from build123d import *

# Parameters (mm, degrees)
SKETCH_1_W          = 56
SKETCH_1_H          = 36
SKETCH_1_R          = 1.6
EXTRUDE_1_DEPTH     = 3
FILLET_1_R          = 3
SKETCH_2_W          = 22
SKETCH_2_H          = 6
SKETCH_2_R          = 1.4
EXTRUDE_2_DEPTH     = 5
SKETCH_3_W          = 22
SKETCH_3_H          = 6
CUT_EXTRUDE_1_DEPTH = 34.660065359
CHAMFER_1_SIZE      = 5


with BuildPart() as part:
    # ｽｹｯﾁ1 → ﾎﾞｽ - 押し出し1 (new body)
    with BuildSketch(Plane(origin=(0, 0, 0), x_dir=(1, 0, 0), z_dir=(0, 1, 0))):
        Rectangle(SKETCH_1_W, SKETCH_1_H)
        with Locations(Location((-25, 15, 0), (0, 0, 270))):
            Circle(SKETCH_1_R, mode=Mode.SUBTRACT)
        with Locations(Location((25, 15, 0), (0, 0, 270))):
            Circle(SKETCH_1_R, mode=Mode.SUBTRACT)
        with Locations(Location((25, -15, 0), (0, 0, 270))):
            Circle(SKETCH_1_R, mode=Mode.SUBTRACT)
        with Locations(Location((-25, -15, 0), (0, 0, 270))):
            Circle(SKETCH_1_R, mode=Mode.SUBTRACT)
    extrude(amount=EXTRUDE_1_DEPTH)

    # ﾌｨﾚｯﾄ1
    fillet_1_edges = [part.edges().sort_by_distance(p)[0] for p in [
        (28, 1.5, 18),
        (-28, 1.5, 18),
        (-28, 1.5, -18),
        (28, 1.5, -18),
    ]]
    fillet(fillet_1_edges, radius=FILLET_1_R)

    # ｽｹｯﾁ2 → ﾎﾞｽ - 押し出し2 (add)
    with BuildSketch(Plane(origin=(0, 3, 0), x_dir=(1, 0, 0), z_dir=(0, 1, 0))):
        with Locations((0, 0.8)):
            Rectangle(SKETCH_2_W, SKETCH_2_H)
        with Locations(Location((-7.5, 0.8, 0), (0, 0, 270))):
            Circle(SKETCH_2_R, mode=Mode.SUBTRACT)
        with Locations(Location((7.5, 0.8, 0), (0, 0, 270))):
            Circle(SKETCH_2_R, mode=Mode.SUBTRACT)
    extrude(amount=EXTRUDE_2_DEPTH)

    # ｽｹｯﾁ3 → ｶｯﾄ - 押し出し1 (cut, through all)
    with BuildSketch(Plane(origin=(0, 3, 0), x_dir=(1, 0, 0), z_dir=(0, 1, 0))):
        with Locations((0, -5.2)):
            Rectangle(SKETCH_3_W, SKETCH_3_H)
    extrude(amount=-CUT_EXTRUDE_1_DEPTH, mode=Mode.SUBTRACT)

    # 面取り1
    chamfer_1_edges = [part.edges().sort_by_distance(p)[0] for p in [
        (-11, 3, -0.8),
        (11, 3, -0.8),
        (0, 3, -3.8),
    ]]
    chamfer(chamfer_1_edges, length=CHAMFER_1_SIZE - 0.0001)  # a hair under: the kernel refuses the full size


solid = part.part
The model under review builds one solid part; all positions refer to its coordinate system, in mm. A direction names the side the tool comes from. Give positions to 0.01 mm unless a question says otherwise; leave off trailing zeros. Loops run counter-clockwise (first coordinate to the right, second up) from the corner with the lowest first, then second, coordinate; pieces in that order, holes last. Notation, with made-up numbers: (-32, 45.5) -> (22, 45.5) arc R24 ccw to (22, 82.5) -> close; hole circle Ø2 at (-10, 4). An arc over 180 degrees is marked (long way). Put each result on its own line as item: value. Start each with the question number.
1. Clearance check with flat-ended pins moving along their axes: P1, Ø3, axis at y = 7, z = 1.5, coming from the -X side; P2, Ø1.5, axis at x = 8.5, z = 9.5, coming from the +Y side. State where each tip first meets the part, or that it passes through.
2. Mouldability with a two-part tool opening along Z and no side actions: class faces 1 (the face through (-13, 6, -2)), 2 (the face through (0, 1, -18)), 3 (the face through (-8.867, 5.465, -1.103)), 4 (the face through (27.1, 1.52, 17.14)) as released by +Z, released by -Z, zero draft, split by the parting line, or undercut.
3. Wall thickness on probe 1 along X at (y, z) = (2.35, -15); probe 2 along Z at (x, y) = (10, 2); probe 3 along X at (y, z) = (4, -2): over which ranges is each line inside the solid? List them lowest first.
4. We need section C-C on z = 6. State the section outline as (x, y) points, then the cut area to 3 significant figures.
5. We need section D-D on z = 14. State the section outline as (x, y) points.
6. For faces 5 (the face through (11, 2, 5)), 6 (the face through (7, 3, -1)), 7 (the face through (13, 6, -2)), list the 3-axis set-ups (+Z, -Z, +X, -X, +Y, -Y) from which the entire face can be reached by the end or side of a thin tool; tool diameter is ignored.
7. We need section B-B on y = 2.25. State the section outline as (x, z) points.
Determined:
1. P1: x = -13.5
1. P2: y = 3
2. face 1: zero draft
2. face 2: released by -Z
2. face 3: undercut
2. face 4: released by +Z
3. probe 1: -28 to -26.6, -23.4 to 23.4, 26.6 to 28
3. probe 2: -18 to 2.2, 8.2 to 18
3. probe 3: -15 to -8.22, -6.78 to 6.78, 8.22 to 15
4. outline: (-28, 0) -> (-11, 0) -> (-11, 3) -> (-28, 3) -> close; (11, 0) -> (28, 0) -> (28, 3) -> (11, 3) -> close
4. area: 102 mm^2
5. outline: (-28, 0) -> (-26.25, 0) -> (-26.25, 3) -> (-28, 3) -> close; (-23.75, 0) -> (23.75, 0) -> (23.75, 3) -> (-23.75, 3) -> close; (26.25, 0) -> (28, 0) -> (28, 3) -> (26.25, 3) -> close
6. face 5: +Y, -Y
6. face 6: +Y
6. face 7: +Z, -Z, +X, +Y
7. outline: (-28, -15) arc R3 ccw to (-25, -18) -> (25, -18) arc R3 ccw to (28, -15) -> (28, 15) arc R3 ccw to (25, 18) -> (-25, 18) arc R3 ccw to (-28, 15) -> close; hole circle Ø3.2 at (-25, -15); hole circle Ø3.2 at (-25, 15); hole (-11, 2.2) -> (11, 2.2) -> (11, 8.2) -> (-11, 8.2) -> close; hole circle Ø3.2 at (25, -15); hole circle Ø3.2 at (25, 15)
